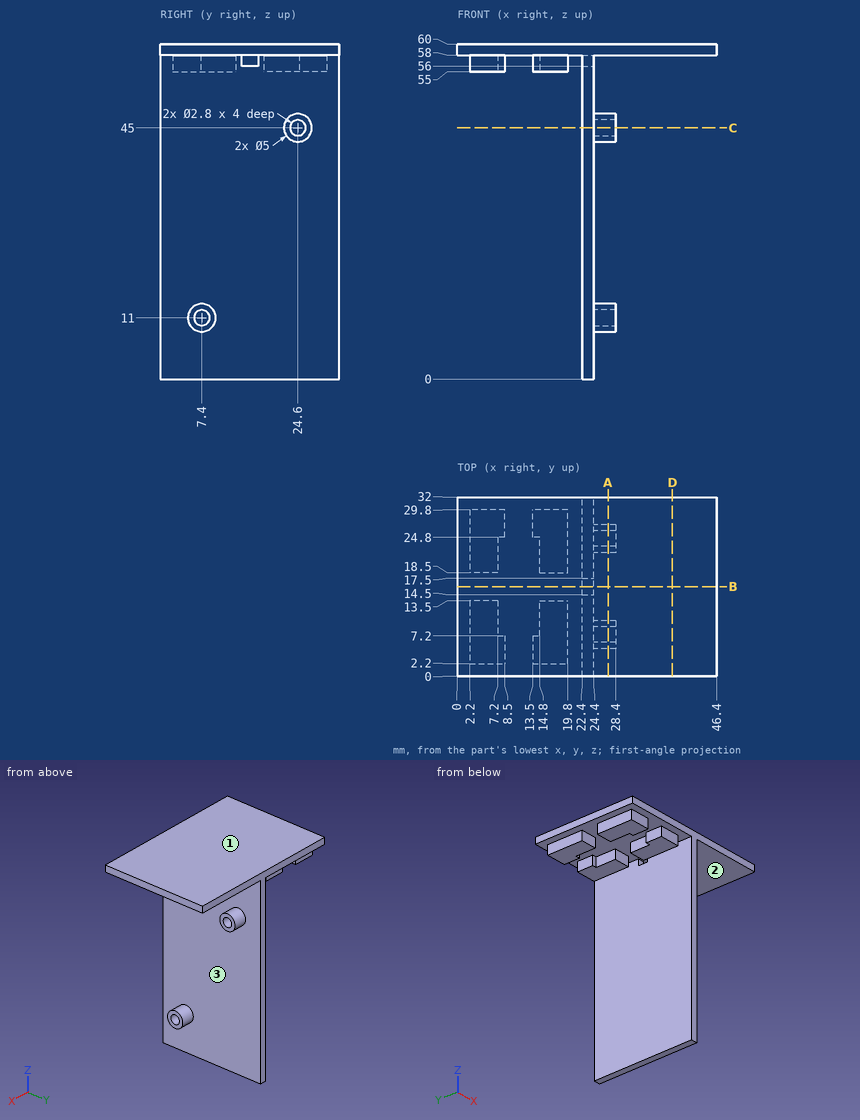
Design review of the part shown in the three views and the two pictorial views. Dimensions are in mm from the part's minimum x, y and z. Give positions to 0.01 mm unless a question says otherwise; leave off trailing zeros. Loops run counter-clockwise (first coordinate to the right, second up) from the corner with the lowest first, then second, coordinate; pieces in that order, holes last. Notation, with made-up numbers: (64.5, -38.5) -> (111.5, -38.5) arc R7 ccw to (111.5, -27.5) -> close; hole circle Ø4 at (70, 89.25). An arc over 180 degrees is marked (long way). Put each result on its own line as item: value. Start each with the question number.
1. Mouldability with a two-part tool opening along X and no side actions: class the marked faces 1, 2 and 3 as released by +X, released by -X, zero draft, split by the parting line, or undercut.
2. We need section C-C on z = 45. State the section outline as (x, y) points, then the cut area to 3 significant figures.
3. We need section B-B on y = 16. State the section outline as (x, z) points, then the cut area to 3 significant figures.
4. We need section A-A on x = 27. State the section outline as (y, z) points.
5. Clearance check with flat-ended pins moving along their axes: P1, Ø3, axis at y = 22.5, z = 27.5, coming from the +X side; P2, Ø3.5, axis at y = 9, z = 56, coming from the -X side; P3, Ø3.5, axis at y = 7.4, z = 11, coming from the +X side. State where each tip first meets the part, or that it passes through.
6. Wall thickness on probe 1 along X at (y, z) = (29, 56.5); probe 2 along Y at (x, z) = (27.25, 45); probe 3 along Z at (x, y) = (25, 7): over which ranges is each line inside the solid? List them lowest first.
7. We need section D-D on x = 38.5. State the section outline as (y, z) points, then the cut area to 3 significant figures.
Determined:
1. face 1: zero draft
1. face 2: undercut
1. face 3: released by +X
2. outline: (22.4, 0) -> (24.4, 0) -> (24.4, 22.1) -> (28.4, 22.1) -> (28.4, 23.2) -> (24.4, 23.2) -> (24.4, 26) -> (28.4, 26) -> (28.4, 27.1) -> (24.4, 27.1) -> (24.4, 32) -> (22.4, 32) -> close
2. area: 72.8 mm^2
3. outline: (0, 58) -> (46.4, 58) -> (46.4, 60) -> (0, 60) -> close; (22.4, 0) -> (24.4, 0) -> (24.4, 56) -> (22.4, 56) -> close
3. area: 205 mm^2
4. outline: (0, 58) -> (32, 58) -> (32, 60) -> (0, 60) -> close; circle Ø5 at (7.4, 11); circle Ø5 at (24.6, 45); hole circle Ø2.8 at (7.4, 11); hole circle Ø2.8 at (24.6, 45)
5. P1: x = 24.4
5. P2: x = 2.2
5. P3: x = 28.4
6. probe 1: 2.2 to 8.5, 13.5 to 19.8, 22.4 to 24.4
6. probe 2: 22.1 to 23.2, 26 to 27.1
6. probe 3: 8.53 to 9.66, 12.34 to 13.47, 58 to 60
7. outline: (0, 58) -> (32, 58) -> (32, 60) -> (0, 60) -> close
7. area: 64.0 mm^2
